Check sheet for the drawn part. Datum: minimum x, y, z corner. Units: mm. A direction names the side the tool comes from. Give positions to 0.01 mm unless a question says otherwise; leave off trailing zeros. Order: outer loops, then holes, each group sorted by start corner. A loop starts at its lowest first (then second) coordinate and runs counter-clockwise, first axis right, second up. Notation, with made-up numbers: (75.25, 74) -> (81.25, 74) arc R32 cw to (81.25, 102) -> close; hole circle Ø3 at (43.5, 8.5). An arc over 180 degrees is marked (long way). Return JSON: item names as keys, results as strings. Group by question number.
(1) Cross-section at C-C on x = 10. Enter the section's corners in (y, z).
(2) Tool access check on the marked faces 4 and 5. Record the directions out of +Z, -Z, +X, -X, +Y, -Y that give a thin tool (end or side, any length) a straight path to the whole face; none if there is none.
(3) Depth check by flat-ended pin: pin 1 Ø3 at (x, z) = (36.5, 1) entering from -Y; pin 2 Ø2 at (x, z) = (33.5, 5) entering from +Y; pin 3 Ø1.5 at (y, z) = (39.5, 2.5) entering from +X. Enter the tip coordinate at first touch or a pass-through.
(4) Cross-section at D-D on z = 2.25. Enter the section's corners in (x, y), then the cut area to 3 significant figures.
(5) Cross-section at B-B on z = 5. Enter the section's corners in (x, y), then the cut area to 3 significant figures.
(6) Release check for a two-part mould opening along Y. For the marked faces 1, 2 and 3 record: pulls with the +Y half, pulls with the -Y half, needs draft (parallel to the pull), parting line crosses it, or undercut.
(7) Thickness scan on line 1 along Y through (x, z) = (25, 5); line 2 along Y through (x, z) = (34.5, 2); line 3 along Y through (x, z) = (43.5, 2.75). Record the ranges inside material, lowest first.
(8) Cross-section at A-A on x = 25. Enter the section's corners in (y, z), then the cut area to 3 significant figures.
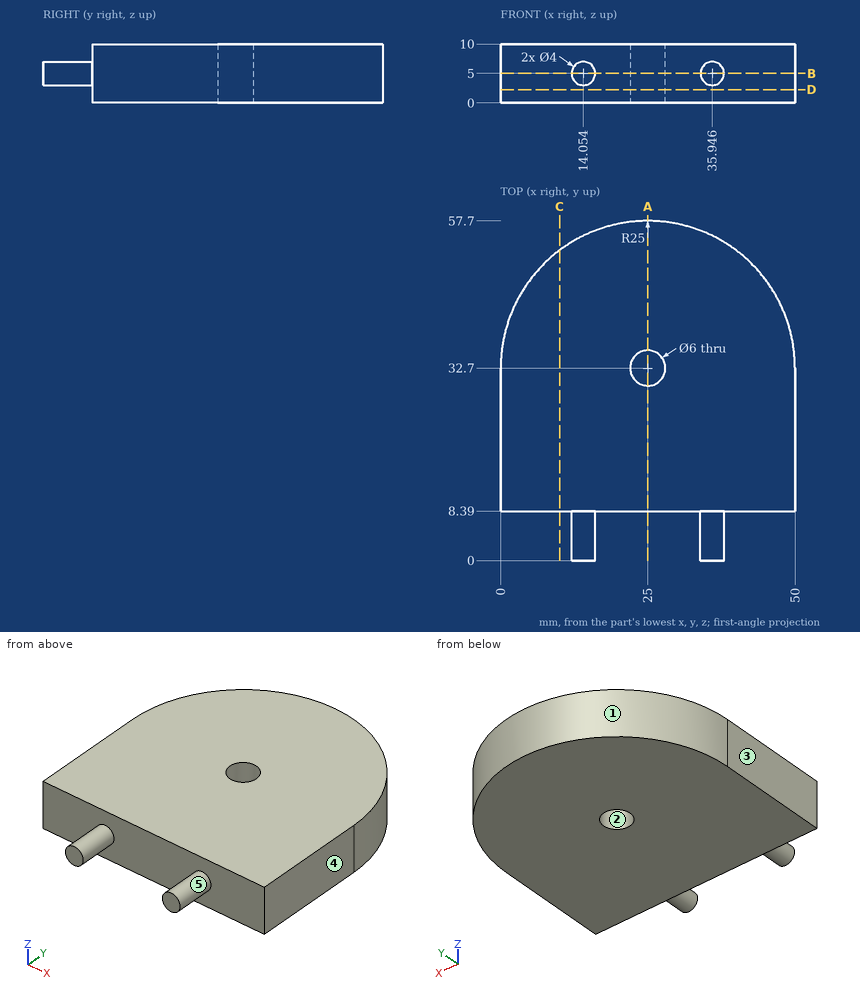
Verdict:
{
 "1": {"outline": "(8.39, 0) -> (52.7, 0) -> (52.7, 10) -> (8.39, 10) -> close"},
 "2": {"face 4": "+Z, -Z, +X, +Y, -Y", "face 5": "-Y"},
 "3": {"pin 1": "y = 8.39", "pin 2": "y = 56.55", "pin 3": "x = 49.26"},
 "4": {"outline": "(0, 8.39) -> (50, 8.39) -> (50, 32.7) arc R25 ccw to (0, 32.7) -> close; hole circle Ø6 at (25, 32.7)", "area": "2,170 mm²"},
 "5": {"outline": "(0, 8.39) -> (12.05, 8.39) -> (12.05, 0) -> (16.05, 0) -> (16.05, 8.39) -> (33.95, 8.39) -> (33.95, 0) -> (37.95, 0) -> (37.95, 8.39) -> (50, 8.39) -> (50, 32.7) arc R25 ccw to (0, 32.7) -> close; hole circle Ø6 at (25, 32.7)", "area": "2,240 mm²"},
 "6": {"face 1": "pulls with the +Y half", "face 2": "undercut", "face 3": "needs draft"},
 "7": {"line 1": "8.39 to 29.7, 35.7 to 57.7", "line 2": "8.39 to 55.82", "line 3": "8.39 to 49.52"},
 "8": {"outline": "(8.39, 0) -> (29.7, 0) -> (29.7, 10) -> (8.39, 10) -> close; (35.7, 0) -> (57.7, 0) -> (57.7, 10) -> (35.7, 10) -> close", "area": "433 mm²"}
}
